The model under review builds one solid part; all positions refer to its coordinate system, in mm. Face numbers are marked on the shaded views. Round coordinates to 2 decimals unless told otherwise and drop trailing zeros. Write each loop counter-clockwise with the first axis right and the second up, starting at its lowest first coordinate (ties: lowest second). Pieces come first, ordered by that corner, then holes. Notation, with made-up numbers: (25, -8.5) -> (78, -8.5) arc R18 cw to (78, 19.5) -> close; hole circle Ø4 at (3, -30.5). An arc over 180 degrees is marked (long way). Answer as a JSON object with one key per item and string values. Group by question number.
1) Insertion check: pin 1 Ø1.5 at (y, z) = (-7.5, 2.5) entering from +X; pin 2 Ø2 at (x, y) = (10.5, -2) entering from -Z; pin 3 Ø2 at (x, y) = (13, -3.5) entering from +Z. Each pin has a flat end and moves straight along its axis. Give the tip position at first contact, or say it passes through.
2) Mouldability with a two-part tool opening along X and no side actions: class the marked faces 1, 2 and 3 as pulls with the +X half, pulls with the -X half, needs draft (parallel to the pull), parting line crosses it, or undercut.
3) We need section A-A, the plane x = 0. Write out the cut boundary in (y, z).
4) To check wall thickness, follow probe 1 along Z at (x, y) = (0, -6); probe 2 along Y at (x, z) = (-18.05, 0); probe 3 along Z at (x, y) = (-1, -1.25). State the ranges of each line that lie inside material, in increasing order. Write a range as [from, to].
5) We need section B-B, the plane z = 0. Write out the cut boundary in (x, y).
6) We need section C-C, the plane y = -7.75. Write out the cut boundary in (x, z), then the cut area to 3 significant figures.
7) We need section D-D, the plane x = -12.5. Write out the cut boundary in (y, z), then the cut area to 3 significant figures.
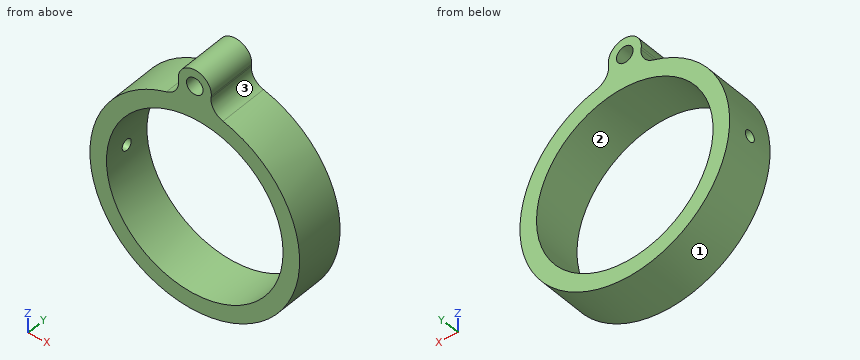
from build123d import *

# Parameters (mm, degrees)
F0_R     = 19
F0_R_2   = 16
F1_DEPTH = 9
F4_R     = 3
F5_DEPTH = 19.001
F6_R     = 1.5
F7_DEPTH = 9
F9_D     = 2
F9_DEPTH = 50
F9_TIP   = 0.600860619


with BuildPart() as f1:
    # F0 (on Front) → F1 (new body)
    with BuildSketch(Plane.XZ):
        Circle(F0_R)
        Circle(F0_R_2, mode=Mode.SUBTRACT)
    extrude(amount=F1_DEPTH)

    # F4 (on Right) → F5 (cut, through all)
    with BuildSketch(Plane.YZ):
        with Locations((-18, 0)):
            Circle(F4_R)
    extrude(amount=-F5_DEPTH, mode=Mode.SUBTRACT)

    # F6 (on face) → F7 (join)
    with BuildSketch(Plane.XZ.offset(9)):
        with BuildLine():
            ThreePointArc((-2.937363317, 21.3901670932), (-3.479735084, 19.4552086117), (-5.1216935171, 18.2966733456))
            ThreePointArc((-5.1216935171, 18.2966733456), (0, 19), (5.1216935171, 18.2966733456))
            ThreePointArc((5.1216935171, 18.2966733456), (3.479735084, 19.4552086117), (2.937363317, 21.3901670932))
            ThreePointArc((2.937363317, 21.3901670932), (2.9582746132, 21.5937605423), (2.993018618, 21.7954544414))
            ThreePointArc((2.993018618, 21.7954544414), (0, 24.9999997616), (-2.993018618, 21.7954544414))
            ThreePointArc((-2.993018618, 21.7954544414), (-2.9582746132, 21.5937605423), (-2.937363317, 21.3901670932))
        make_face()
        with Locations((0, 21.9999998808)):
            Circle(F6_R, mode=Mode.SUBTRACT)
        with BuildLine():
            ThreePointArc((-2.993018618, 21.7954544414), (-2.9721073218, 21.5918609923), (-2.937363317, 21.3901670932))
            ThreePointArc((-2.937363317, 21.3901670932), (-2.9582746132, 21.5937605423), (-2.993018618, 21.7954544414))
        make_face()
        with BuildLine():
            ThreePointArc((2.993018618, 21.7954544414), (2.9582746132, 21.5937605423), (2.937363317, 21.3901670932))
            ThreePointArc((2.937363317, 21.3901670932), (2.9721073218, 21.5918609923), (2.993018618, 21.7954544414))
        make_face()
    extrude(amount=-F7_DEPTH)

    # F9 (one way)
    with BuildSketch(Plane.YZ):
        with Locations((-4.5, 0)):
            Circle(F9_D / 2)
    extrude(amount=-F9_DEPTH, mode=Mode.SUBTRACT)
    with Locations(Plane.YZ):
        with Locations((-4.5, 0)):
            with Locations((0, 0, -(F9_DEPTH + F9_TIP / 2))):  # 118° drill point
                Cone(0, F9_D / 2, F9_TIP, mode=Mode.SUBTRACT)


solid = f1.part
Here are the results:
{
 "1": {"pin 1": "stops at x = 18.92", "pin 2": "stops at z = -16.45", "pin 3": "stops at z = 14.73"},
 "2": {"face 1": "parting line crosses it", "face 2": "undercut", "face 3": "pulls with the +X half"},
 "3": {"outline": "(-9, -19) -> (0, -19) -> (0, -16) -> (-9, -16) -> close; (-9, 16) -> (0, 16) -> (0, 20.5) -> (-9, 20.5) -> close; (-9, 23.5) -> (0, 23.5) -> (0, 25) -> (-9, 25) -> close"},
 "4": {"probe 1": "z = [-19, -16], [16, 20.5], [23.5, 25]", "probe 2": "y = [-9, -5.5], [-3.5, 0]", "probe 3": "z = [-18.97, -15.97], [15.97, 20.88], [23.12, 24.83]"},
 "5": {"outline": "(-19, -9) -> (-16, -9) -> (-16, -5.5) -> (-19, -5.5) -> close; (-19, -3.5) -> (-16, -3.5) -> (-16, 0) -> (-19, 0) -> close; (16, -9) -> (19, -9) -> (19, 0) -> (16, 0) -> close"},
 "6": {"outline": "(-5.12, 18.3) arc R19 ccw (long way) to (5.12, 18.3) arc R3 cw to (2.94, 21.39) arc R3 ccw (long way) to (-2.94, 21.39) arc R3 cw to start; hole circle Ø32 at (0, 0); hole circle Ø3 at (0, 22)", "area": "357 mm^2"},
 "7": {"outline": "(-9, -14.31) -> (0, -14.31) -> (0, -9.99) -> (-9, -9.99) -> close; (-9, 9.99) -> (0, 9.99) -> (0, 14.31) -> (-9, 14.31) -> close", "area": "77.8 mm^2"}
}
